```python
from build123d import *

# Parameters (mm, degrees)
F1_DEPTH  = 78.6
F4_DEPTH  = 72.6
F5_W      = 18
F5_H      = 72.6
F6_DEPTH  = 5
F8_DEPTH  = 5
F10_DEPTH = 5
F12_DEPTH = 13
F13_R     = 5
F14_R     = 2
F15_R     = 1.25
F16_DEPTH = 25
F17_W     = 10.3
F17_H     = 3
F18_DEPTH = 42.5
F20_R     = 1.95
F21_DEPTH = 4
F22_SIZE  = 2
F23_R     = 2


with BuildPart() as f1:
    # F0 (on Front) → F1 (new body)
    with BuildSketch(Plane.XZ):
        Polygon((-50, 0), (0, 0), (0, 60), (-15, 60), (-50, 30), align=None)
    extrude(amount=F1_DEPTH)

    # F3 (on offset) → F4 (cut)
    with BuildSketch(Plane.XZ.offset(3)):
        Polygon((-47, 3), (0, 3), (0, 36.5), (-3, 36.5), (-3, 57), (-13.8902277714, 57), (-47, 28.6201952326), align=None)
    extrude(amount=F4_DEPTH, mode=Mode.SUBTRACT)

    # F5 (on face) → F6 (cut)
    with BuildSketch(Plane(origin=(0, 0, 0), x_dir=(1, 0, 0), z_dir=(0, 0, -1))):
        with Locations((-9, 39.3)):
            Rectangle(F5_W, F5_H)
    extrude(amount=-F6_DEPTH, mode=Mode.SUBTRACT)

    # F7 (on Front) → F8 (cut)
    with BuildSketch(Plane.XZ):
        with BuildLine():
            Line((-6.5, 24), (0, 24))
            Line((0, 24), (0, 28))
            Line((0, 28), (-6.5, 28))
            ThreePointArc((-6.5, 28), (-7.5606601718, 27.5606601718), (-8, 26.5))
            Line((-8, 26.5), (-8, 25.5))
            ThreePointArc((-8, 25.5), (-7.5606601718, 24.4393398282), (-6.5, 24))
        make_face()
    extrude(amount=F8_DEPTH, mode=Mode.SUBTRACT)

    # F9 (on face) → F10 (cut)
    with BuildSketch(Plane.XZ.offset(78.6)):
        with BuildLine():
            Line((-8, 24), (0, 24))
            Line((0, 24), (0, 31))
            Line((0, 31), (-8, 31))
            ThreePointArc((-8, 31), (-10.1213203436, 30.1213203436), (-11, 28))
            Line((-11, 28), (-11, 27))
            ThreePointArc((-11, 27), (-10.1213203436, 24.8786796564), (-8, 24))
        make_face()
    extrude(amount=-F10_DEPTH, mode=Mode.SUBTRACT)

    # F11 (on face) → F12 (join)
    with BuildSketch(Plane.XY.offset(60)):
        Polygon((-4, -24.3), (-4, -39.3), (-4, -54.3), (0, -54.3), (0, -39.3), (0, -24.3), align=None)
    extrude(amount=F12_DEPTH)

    # F13
    f13_edges = [f1.edges().sort_by_distance(p)[0] for p in [
        (-2, -54.3, 73),
        (-2, -24.3, 73),
        (-15, -39.3, 60),
        (-50, -39.3, 30),
        (-50, -39.3, 0),
    ]]
    fillet(f13_edges, radius=F13_R)

    # F14
    f14_edges = [f1.edges().sort_by_distance(p)[0] for p in [
        (-4, -54.3, 64),
        (-32.329147, 0, 45.146446),
        (-32.329147, -78.6, 45.146446),
    ]]
    fillet(f14_edges, radius=F14_R)

    # F15 (on face) → F16 (cut)
    with BuildSketch(Plane.YZ):
        with Locations((-39.3, 68.5)):
            Circle(F15_R)
    extrude(amount=-F16_DEPTH, mode=Mode.SUBTRACT)

    # F17 (on face) → F18 (join)
    with BuildSketch(Plane.YZ.offset(-47)):
        with Locations((-8.15, 4.5)):
            Rectangle(F17_W, F17_H)
        with Locations((-70.45, 4.5)):
            Rectangle(F17_W, F17_H)
    extrude(amount=F18_DEPTH)

    # F20 (on offset) → F21 (join)
    with BuildSketch(Plane.XY.offset(3)):
        with Locations((-10.5, -9.3)):
            Circle(F20_R)
        with Locations((-10.5, -69.3)):
            Circle(F20_R)
    extrude(amount=-F21_DEPTH)

    # F22
    f22_edges = [f1.edges().sort_by_distance(p)[0] for p in [
        (-3, -39.3, 36.5),
    ]]
    chamfer(f22_edges, length=F22_SIZE)

    # F23
    f23_edges = [f1.edges().sort_by_distance(p)[0] for p in [
        (-47, -8.15, 6),
        (-47, -13.3, 4.5),
        (-32.5, -13.3, 3),
        (-47, -70.45, 6),
        (-47, -65.3, 4.5),
        (-32.5, -65.3, 3),
        (-25.75, -75.6, 6),
        (-25.75, -3, 6),
        (-47, -3, 17.310098),
        (-30.445114, -3, 42.810098),
        (-47, -39.3, 28.620195),
        (-47, -75.6, 17.310098),
        (-30.445114, -75.6, 42.810098),
        (-13.890228, -39.3, 57),
        (-8.445114, -3, 57),
        (-8.445114, -75.6, 57),
    ]]
    fillet(f23_edges, radius=F23_R)


solid = f1.part
```
Verification items for the finished model (mm, model axes). A direction names the side the tool comes from. Give positions to 0.01 mm unless a question says otherwise; leave off trailing zeros. Write each loop counter-clockwise with the first axis right and the second up, starting at its lowest first coordinate (ties: lowest second). Pieces come first, ordered by that corner, then holes. Notation, with made-up numbers: M 66.5,73 L 123.5,73 A17 cw 123.5,79 Z; hole C 77.5,77 d6. An arc over 180 degrees is marked long. One line per question, with ' | ' between items.
1) Thickness scan on line 1 along Y through (x, z) = (-12, 11.5); line 2 along Z through (x, y) = (-12.5, -6.5); line 3 along X through (y, z) = (-34, 14). Record the ranges inside material, lowest first. Write a range as [from, to].
Result:
line 1: y = [-78.6, -75.6], [-3, 0] | line 2: z = [3, 6], [57, 60] | line 3: x = [-50, -47]
2) Gauge pin test, flat ends, axial feed: pin 1 Ø5 at (x, y) = (-12, -26.5) entering from -Z; pin 2 Ø4 at (y, z) = (-71.5, 4.5) entering from +X; pin 3 Ø3.5 at (x, y) = (-4, -1) entering from +Z. Record the tip position at first contact, or that the pin passes through.
Result:
pin 1: stops at z = 56.48 | pin 2: stops at x = -4.5 | pin 3: stops at z = 60
3) Mould release check, pull along X, two halves, no side actions. Record for faces 6 (the flat face through (-25, -70, 6)), 7 (the flat face through (0, -39, 50)), 8 (the flat face through (-2, -38.8, 37.5)), 9 (the flat face through (-32.106, -38.778, 45.338)): released by +X, released by -X, zero draft, split by the parting line, or undercut.
Result:
face 6: zero draft | face 7: released by +X | face 8: undercut | face 9: released by -X
4) Section check B-B on z = 10. Enter the section's corners in (x, y).
Result:
outline: M -50,-76.6 A2 ccw -48,-78.6 L 0,-78.6 L 0,-75.6 L -45,-75.6 A2 cw -47,-73.6 L -47,-5 A2 cw -45,-3 L 0,-3 L 0,0 L -48,0 A2 ccw -50,-2 Z
5) Set-up check for faces 1 (the flat face through (-4.5, -71, 4)), 2 (the cylindrical face through (-10.14, -77.12, 24.9)), 3 (the cylindrical face through (-32.3, -13.87, 3.6)), 4 (the cylindrical face through (-30.21, -3.57, 42.22)), 5 (the flat face through (-11, -7, 3)): record each of +Z, -Z, +X, -X, +Y, -Y from which the full face is reachable in a straight line by a thin tool's end or side.
Result:
face 1: -Z, +X | face 2: +X, -Y | face 3: +X | face 4: none | face 5: -Z
6) Section check A-A on y = -69.3. Enter the section's corners in (x, z).
Result:
outline: M -50,5 A5 ccw -45,0 L -18,0 L -18,3 L -12.45,3 L -12.45,-1 L -8.55,-1 L -8.55,3 L -4.5,3 L -4.5,6 L -45,6 A2 cw -47,8 L -47,27.7 A2 cw -46.3,29.22 L -14.45,56.52 A2 cw -13.15,57 L -3,57 L -3,38.5 L -1,36.5 L 0,36.5 L 0,60 L -13.15,60 A5 ccw -16.4,58.8 L -48.25,31.5 A5 ccw -50,27.7 Z
